Design review of the part built by this model. Coordinates are the model's own, in mm. A direction names the side the tool comes from. Coordinates: 2 decimals unless noted, no trailing zeros. Loops run counter-clockwise (first coordinate to the right, second up) from the corner with the lowest first, then second, coordinate; pieces in that order, holes last. Notation, with made-up numbers: (86.5, -3) - (93.5, -3) arc R17 cw to (93.5, 14) - close; hole circle Ø8 at (51, 16). An arc over 180 degrees is marked (long way). Answer in a Markdown table with one row per item. Add a question column.
(1) Clearance check with a flat-ended pin moving along its axis: pin 1 (6 mm diameter, centred on x = 5, y = -8.66, fed in from +Z). State where the tip first meets the part, or that it passes through.
(2) We need section C-C, the plane z = 7. Write out the cut boundary in (x, y), plus the area to 3 significant figures.
(3) For faces 4 (the face through (5.93, -2.27, 2.46)), 5 (the face through (-66.385, 9.411, 6.479)), list the 3-axis set-ups (+Z, -Z, +X, -X, +Y, -Y) from which the entire face can be reached by the end or side of a thin tool; tool diameter is ignored.
(4) We need section B-B, the plane z = 1.5. Write out the cut boundary in (x, y).
(5) We need section A-A, the plane y = 0. Write out the cut boundary in (x, z), plus the area to 3 significant figures.
(6) We need section D-D, the plane x = -24.5. Write out the cut boundary in (y, z), plus the area to 3 significant figures.
(7) The part is to be moulded in two halves that separate along X. For faces 1 (the face through (-64.93, 2.27, 2.46)), 2 (the face through (-0.54, -2.44, 2.46)), 3 (the face through (-29, 0, 0)), say which applies: released by +X, released by -X, zero draft, split by the parting line, or undercut.
(8) To check wall thickness, follow L1, parallel to X at y = -0.25, z = 3; L2, parallel to X at y = 1, z = 4.5; L3, parallel to Y at x = -64, z = 5.5. State the ranges of each line that lie inside material, in increasing order. Write a range as [from, to].
from build123d import *

# Parameters (mm, degrees)
SKETCH2_R           = 2.5
BOSS_EXTRUDE1_DEPTH = 5
SKETCH4_R           = 2.5
SKETCH4_R_2         = 0.5
BOSS_EXTRUDE3_DEPTH = 8


with BuildPart() as part:
    # Sketch2 → Boss-Extrude1 (new body)
    with BuildSketch(Plane.XY):
        with BuildLine():
            Line((-63.463622529, 12.624128305), (0.536377471, 3.963874268))
            ThreePointArc((0.536377471, 3.963874268), (2.228263621, 3.321873152), (3.464101615, 2))
            Line((3.464101615, 2), (8.464101615, -6.660254038))
            ThreePointArc((8.464101615, -6.660254038), (8.321873152, -10.888517659), (4.463622529, -12.624128305))
            Line((4.463622529, -12.624128305), (-59.536377471, -3.963874268))
            ThreePointArc((-59.536377471, -3.963874268), (-61.228263621, -3.321873152), (-62.464101615, -2))
            Line((-62.464101615, -2), (-67.464101615, 6.660254038))
            ThreePointArc((-67.464101615, 6.660254038), (-67.321873152, 10.888517659), (-63.463622529, 12.624128305))
        make_face()
        with Locations((-59, 0)):
            Circle(SKETCH2_R, mode=Mode.SUBTRACT)
        with Locations((-64, 8.660254038)):
            Circle(SKETCH2_R, mode=Mode.SUBTRACT)
        Circle(SKETCH2_R, mode=Mode.SUBTRACT)
        with Locations((5, -8.660254038)):
            Circle(SKETCH2_R, mode=Mode.SUBTRACT)
    extrude(amount=BOSS_EXTRUDE1_DEPTH)

    # Sketch4 → Boss-Extrude3 (add)
    with BuildSketch(Plane(origin=(0, 0, 0), x_dir=(-1, 0, 0), z_dir=(0, 0, -1))):
        with Locations((64, 8.660254038)):
            Circle(SKETCH4_R)
        with Locations((64, 8.660254038)):
            Circle(SKETCH4_R_2, mode=Mode.SUBTRACT)
    extrude(amount=-BOSS_EXTRUDE3_DEPTH)


solid = part.part
Responses:
| question | item | result |
|---|---|---|
| 1 | pin 1 | stops at z = 5 |
| 2 | outline | circle Ø5 at (-64, 8.66); hole circle Ø1 at (-64, 8.66) |
| 2 | area | 18.8 mm2 |
| 3 | face 4 | +Z, -Z, +X, +Y |
| 3 | face 5 | +Z |
| 4 | outline | (-67.46, 6.66) - (-62.46, -2) arc R4 ccw to (-59.54, -3.96) - (4.46, -12.62) arc R4 ccw to (8.46, -6.66) - (3.46, 2) arc R4 ccw to (0.54, 3.96) - (-63.46, 12.62) arc R4 ccw to start; hole circle Ø1 at (-64, 8.66); hole circle Ø5 at (-59, 0); hole circle Ø5 at (0, 0); hole circle Ø5 at (5, -8.66) |
| 5 | outline | (-63.62, 0) - (-61.5, 0) - (-61.5, 5) - (-63.62, 5) - close; (-56.5, 0) - (-2.5, 0) - (-2.5, 5) - (-56.5, 5) - close; (2.5, 0) - (4.62, 0) - (4.62, 5) - (2.5, 5) - close |
| 5 | area | 291 mm2 |
| 6 | outline | (-8.7, 0) - (7.35, 0) - (7.35, 5) - (-8.7, 5) - close |
| 6 | area | 80.3 mm2 |
| 7 | face 1 | released by -X |
| 7 | face 2 | undercut |
| 7 | face 3 | zero draft |
| 8 | L1 | x = [-63.47, -61.49], [-56.51, -2.49], [2.49, 4.76] |
| 8 | L2 | x = [-64.2, -61.29], [-56.71, -2.29], [2.29, 4.04] |
| 8 | L3 | y = [6.16, 8.16], [9.16, 11.16] |
